from build123d import *

# Parameters (mm, degrees)
F0_R     = 9.422472
F1_DEPTH = 19.05
F2_DEPTH = 25.4


with BuildPart() as f1:
    # F0 (on Front) → F1 (new body)
    with BuildSketch(Plane.XZ):
        with BuildLine():
            ThreePointArc((-16.764912, 53.948052), (0, 37.183141), (16.764912, 53.948052))
            ThreePointArc((16.764912, 53.948052), (0, 70.712964), (-16.764912, 53.948052))
        make_face()
        with Locations((0, 53.948052)):
            Circle(F0_R, mode=Mode.SUBTRACT)
        with BuildLine():
            ThreePointArc((-16.764912, 0), (0, 16.764912), (16.764912, 0))
            Line((16.764912, 0), (16.764912, 53.948052))
            ThreePointArc((16.764912, 53.948052), (0, 37.183141), (-16.764912, 53.948052))
            Line((-16.764912, 53.948052), (-16.764912, 0))
        make_face()
        with BuildLine():
            ThreePointArc((-16.764912, 0), (0, -16.764912), (16.764912, 0))
            ThreePointArc((16.764912, 0), (0, 16.764912), (-16.764912, 0))
        make_face()
        Circle(F0_R, mode=Mode.SUBTRACT)
    extrude(amount=F1_DEPTH)

    # F0 (on Front) → F2 (join)
    with BuildSketch(Plane.XZ):
        with BuildLine():
            ThreePointArc((-16.764912, 0), (0, -16.764912), (16.764912, 0))
            ThreePointArc((16.764912, 0), (0, 16.764912), (-16.764912, 0))
        make_face()
        Circle(F0_R, mode=Mode.SUBTRACT)
    extrude(amount=-F2_DEPTH)

    # F3: F1 across face


with BuildPart() as f1_1:
    add(f1.part)
    add(f1.part.mirror(Plane(origin=(0, 25.4, 0), x_dir=(1, 0, 0), z_dir=(0, 1, 0))))


solid = f1_1.part
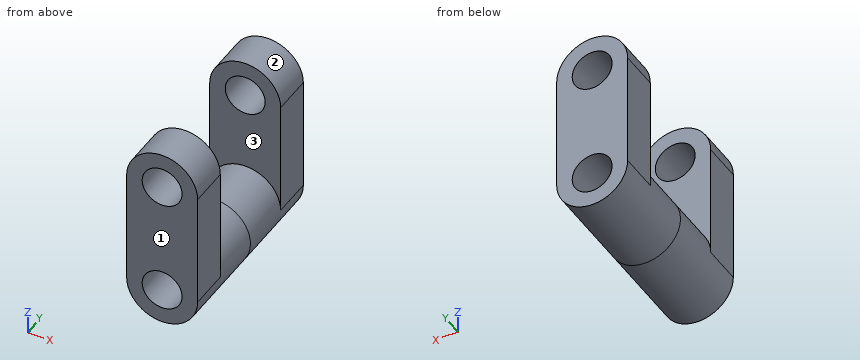
The model under review builds one solid part; all positions refer to its coordinate system, in mm. Face numbers are marked on the shaded views. Give positions to 0.01 mm unless a question says otherwise; leave off trailing zeros. Loops run counter-clockwise (first coordinate to the right, second up) from the corner with the lowest first, then second, coordinate; pieces in that order, holes last. Notation, with made-up numbers: (-14, 22.25) -> (-4, 22.25) arc R30 ccw to (-4, 50.25) -> close; hole circle Ø7 at (67.5, 78). An arc over 180 degrees is marked (long way). Answer as a JSON object with one key per item and string values. Group by question number.
Q1. Take a section at C-C (y = 58). Write out the cut boundary in (x, z).
Q2. Take a section at A-A (z = 34). Write out the cut boundary in (x, y).
Q3. Insertion check: pin 1 (1.5 mm diameter, centred on y = 20, z = 13.5, fed in from +X); pin 2 (1 mm diameter, centred on x = 5, y = 49, fed in from -Z); pin 3 (2 mm diameter, centred on y = 38.5, z = -7.5, fed in from -X); pin 4 (15 mm diameter, centred on x = 0, z = 0, fed in from +Y). Each pin has a flat end and moves straight along its axis. Give the tip position at first contact, or say it passes through.
Q4. Take a section at B-B (x = 0). Write out the cut boundary in (y, z), plus the area to 3 significant figures.
Q5. Take a section at D-D (x = 7.5). Write out the cut boundary in (y, z), plus the area to 3 significant figures.
Q6. Wall thickness on line 1 along Z through (x, y) = (0, -11.75); line 2 along Y through (x, z) = (-3, 20); line 3 along Z through (x, y) = (0, 9.25): over which ranges is each line inside the solid? List them lowest first.
Q7. Draft analysis for pull direction Y (two halves, no side actions). For the marked faces 1, 2 and 3, state which applies: pulls with the +Y half, pulls with the -Y half, needs draft (parallel to the pull), parting line crosses it, or undercut.
Answer below:
{
 "1": {"outline": "(-16.76, 0) arc R16.76 ccw to (16.76, 0) -> (16.76, 53.95) arc R16.76 ccw to (-16.76, 53.95) -> close; hole circle Ø18.84 at (0, 0); hole circle Ø18.84 at (0, 53.95)"},
 "2": {"outline": "(-16.76, -19.05) -> (16.76, -19.05) -> (16.76, 0) -> (-16.76, 0) -> close; (-16.76, 50.8) -> (16.76, 50.8) -> (16.76, 69.85) -> (-16.76, 69.85) -> close"},
 "3": {"pin 1": "stops at x = 10.89", "pin 2": "stops at z = -16.15", "pin 3": "stops at x = -15.45", "pin 4": "passes through"},
 "4": {"outline": "(-19.05, -16.76) -> (69.85, -16.76) -> (69.85, -9.42) -> (-19.05, -9.42) -> close; (-19.05, 9.42) -> (69.85, 9.42) -> (69.85, 44.53) -> (50.8, 44.53) -> (50.8, 16.76) -> (0, 16.76) -> (0, 44.53) -> (-19.05, 44.53) -> close; (-19.05, 63.37) -> (0, 63.37) -> (0, 70.71) -> (-19.05, 70.71) -> close; (50.8, 63.37) -> (69.85, 63.37) -> (69.85, 70.71) -> (50.8, 70.71) -> close", "area": "2,640 mm2"},
 "5": {"outline": "(-19.05, -14.99) -> (69.85, -14.99) -> (69.85, -5.7) -> (-19.05, -5.7) -> close; (-19.05, 5.7) -> (69.85, 5.7) -> (69.85, 48.24) -> (50.8, 48.24) -> (50.8, 14.99) -> (0, 14.99) -> (0, 48.24) -> (-19.05, 48.24) -> close; (-19.05, 59.65) -> (0, 59.65) -> (0, 68.94) -> (-19.05, 68.94) -> close; (50.8, 59.65) -> (69.85, 59.65) -> (69.85, 68.94) -> (50.8, 68.94) -> close", "area": "3,270 mm2"},
 "6": {"line 1": "z = -16.76 to -9.42, 9.42 to 44.53, 63.37 to 70.71", "line 2": "y = -19.05 to 0, 50.8 to 69.85", "line 3": "z = -16.76 to -9.42, 9.42 to 16.76"},
 "7": {"face 1": "pulls with the -Y half", "face 2": "needs draft", "face 3": "undercut"}
}
